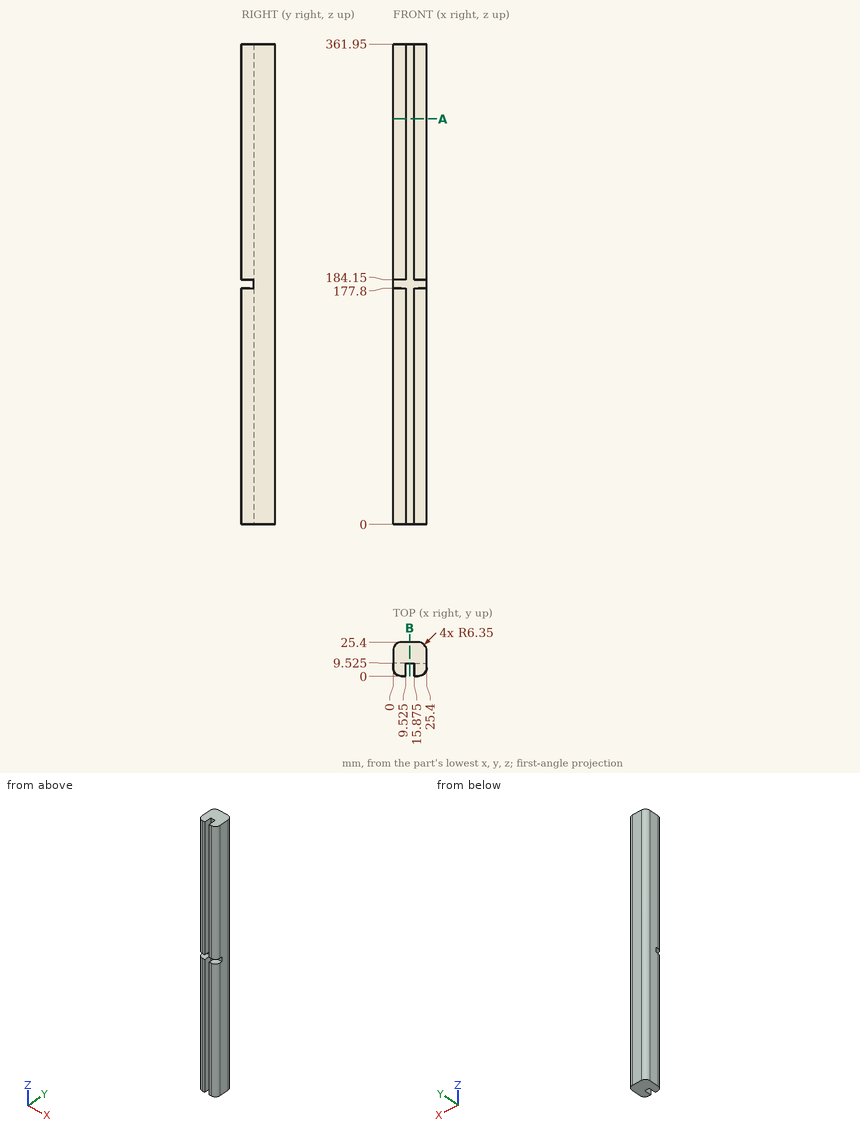
Design review of the part shown in the three views and the two pictorial views. Dimensions are in mm from the part's minimum x, y and z. Round coordinates to 2 decimals unless told otherwise and drop trailing zeros. Loops run counter-clockwise (first coordinate to the right, second up) from the corner with the lowest first, then second, coordinate; pieces in that order, holes last. Notation, with made-up numbers: (7.25, 72) -> (56.25, 72) arc R29 ccw to (56.25, 103) -> close; hole circle Ø7 at (-15.5, -36). An arc over 180 degrees is marked (long way). Answer as a JSON object with one key per item and string values. Group by question number.
1) For line 1 (Z direction, x = 23, y = 6); line 2 (X direction, y = 8.75, z = 233) (3 decimals); line 3 (X direction, y = 19.25, z = 56.5), list the stretches that pass through material, from the lowest coordinate up. Write a range as [from, to].
2) For pin 1 Ø3 at (y, z) = (3.5, 300.5) entering from -X; pin 2 Ø5 at (y, z) = (3.5, 54.5) entering from -X, all flat-tipped, find the tip position at first contact; note any pin that passes through.
3) We need section A-A on z = 305.5. Write out the cut boundary in (x, y) (3 decimals).
4) We need section B-B on x = 12.5. Write out the cut boundary in (y, z) (3 decimals), then the cut area to 3 significant figures.
Result set:
{
 "1": {"line 1": "[0, 177.8], [184.15, 361.95]", "line 2": "[0, 9.525], [15.875, 25.4]", "line 3": "[0, 25.4]"},
 "2": {"pin 1": "x = 0.15", "pin 2": "x = 0.01"},
 "3": {"outline": "(0, 6.35) arc R6.35 ccw to (6.35, 0) -> (9.525, 0) -> (9.525, 9.525) -> (15.875, 9.525) -> (15.875, 0) -> (19.05, 0) arc R6.35 ccw to (25.4, 6.35) -> (25.4, 19.05) arc R6.35 ccw to (19.05, 25.4) -> (6.35, 25.4) arc R6.35 ccw to (0, 19.05) -> close"},
 "4": {"outline": "(9.525, 0) -> (25.4, 0) -> (25.4, 361.95) -> (9.525, 361.95) -> close", "area": "5,750 mm²"}
}
